Design review of the part built by this model. Coordinates are the model's own, in mm. A direction names the side the tool comes from. Coordinates: 2 decimals unless noted, no trailing zeros. Loops run counter-clockwise (first coordinate to the right, second up) from the corner with the lowest first, then second, coordinate; pieces in that order, holes last. Notation, with made-up numbers: (-31.5, 79.25) -> (-5.5, 79.25) arc R26 cw to (-5.5, 96.25) -> close; hole circle Ø3 at (64, -29). An arc over 180 degrees is marked (long way). Use one line per item in the form item = value. Start each with the question number.
1. For pin 1 (2 mm diameter, centred on x = 1, z = 27.5, fed in from -Y); pin 2 (1 mm diameter, centred on x = 0, y = 0, fed in from -Z); pin 3 (2 mm diameter, centred on x = -1.5, z = 53.5, fed in from +Y), all flat-tipped, find the tip position at first contact; note any pin that passes through.
2. Consider section A-A (x = 0). State the section outline as (y, z) points, then the cut area to 3 significant figures.
3. Machinability: for faces 4 (the face through (2.4, -4.5, 3)), 5 (the face through (0, -1, -6)), which of the approach directions +Z, -Z, +X, -X, +Y, -Y give a long, thin tool a straight path to every point of the face, cutting with its end or side? Answer none if there is none.
4. Consider section D-D (z = 55). State the section outline as (x, y) points, then the cut area to 3 significant figures.
5. Wall thickness on line 1 (Y direction, x = 0, z = -4.5); line 2 (Y direction, x = 0.75, z = -5); line 3 (Y direction, x = 0, z = 96): over which ranges is each line inside the solid? List them lowest first. Write a range as from..to.
6. The part is to be moulded in two halves that separate along X. For faces 1 (the face through (0, 0, 3)), 2 (the face through (-1.5, 0.07, 59.6)), 3 (the face through (3.3, -1.1, 0)), say which applies: released by +X, released by -X, zero draft, split by the parting line, or undercut.
7. Consider section C-C (z = -5.5). State the section outline as (x, y) points, then the cut area to 3 significant figures.
from build123d import *

# Parameters (mm, degrees)
ESQUISSE1_R             = 8.5
BOSS_EXTRU_1_DEPTH      = 10
ESQUISSE2_R             = 2.5
BOSS_EXTRU_2_DEPTH      = 157
ECHELLE2_SCALE          = 0.6
ESQUISSE5_R             = 3.25
BOSS_EXTRU_4_DEPTH      = 14
ESQUISSE6_R             = 1
ENL_V_MAT_EXTRU_1_DEPTH = 17
D_ME1_FACE_RADIUS       = 1.5
D_ME1_HEIGHT            = 1.5


with BuildPart() as part:
    # Esquisse1 → Boss.-Extru.1 (new body)
    with BuildSketch(Plane.XY):
        Circle(ESQUISSE1_R)
    extrude(amount=BOSS_EXTRU_1_DEPTH)

    # Esquisse2 → Boss.-Extru.2 (add)
    with BuildSketch(Plane.XY.offset(10)):
        Circle(ESQUISSE2_R)
    extrude(amount=BOSS_EXTRU_2_DEPTH)


with BuildPart() as part_1:
    # Echelle2: scaled about (0, 0, 0)
    add(part.part.scale(ECHELLE2_SCALE))

    # Esquisse5 → Boss.-Extru.4 (add)
    with BuildSketch(Plane(origin=(0, 0, 0), x_dir=(-1, 0, 0), z_dir=(0, 0, -1))):
        with Locations(Location((0, 0, 0), (0, 0, 180))):
            Circle(ESQUISSE5_R)
    extrude(amount=BOSS_EXTRU_4_DEPTH)

    # Esquisse6 → Enlèv. mat.-Extru.1 (cut)
    with BuildSketch(Plane(origin=(0, 0, -14), x_dir=(-1, 0, 0), z_dir=(0, 0, -1))):
        Circle(ESQUISSE6_R)
    extrude(amount=-ENL_V_MAT_EXTRU_1_DEPTH, mode=Mode.SUBTRACT)

    # Esquisse8 → Révolution1 (revolve)
    with BuildSketch(Plane(origin=(0, 0, 0), x_dir=(1, 0, 0), z_dir=(0, 1, 0)), mode=Mode.PRIVATE) as r_volution1_sk:
        Polygon((5.1, -6), (0, -6), (0, -26), align=None)
    revolve(r_volution1_sk.sketch.rotate(Axis((0, 0, 6), (0, 0, 1)), 180), axis=Axis((0, 0, 6), (0, 0, 1)))

    # Dôme1: a dome of height H over a round flat face of radius A is a cap of a sphere of radius (A * A + H * H) / (2 * H)
    d_me1_r = (D_ME1_FACE_RADIUS * D_ME1_FACE_RADIUS + D_ME1_HEIGHT * D_ME1_HEIGHT) / (2 * D_ME1_HEIGHT)
    d_me1_base = Plane((0, 0, 100.2), z_dir=(0, 0, 1))
    with Locations(d_me1_base.offset(D_ME1_HEIGHT - d_me1_r)):
        d_me1_ball = Sphere(d_me1_r, mode=Mode.PRIVATE)
    add(split(d_me1_ball, bisect_by=d_me1_base, keep=Keep.TOP, mode=Mode.PRIVATE))


solid = part_1.part
Geometry check:
q1.pin_1 = -1.5
q1.pin_2 = 3
q1.pin_3 = 1.41
q2.outline = (-5.1, 0) -> (-3.25, 0) -> (-3.25, -14) -> (-1, -14) -> (-1, 3) -> (1, 3) -> (1, -14) -> (3.25, -14) -> (3.25, 0) -> (5.1, 0) -> (5.1, 6) -> (1.5, 20.12) -> (1.5, 100.2) arc R1.5 ccw to (-1.5, 100.2) -> (-1.5, 20.12) -> (-5.1, 6) -> close
q2.area = 455 mm²
q3.face_4 = +Z, -Z
q3.face_5 = -Z
q4.outline = circle Ø3 at (0, 0)
q4.area = 7.07 mm²
q5.line_1 = -3.25..-1, 1..3.25
q5.line_2 = -3.16..-0.66, 0.66..3.16
q5.line_3 = -1.5..1.5
q6.face_1 = undercut
q6.face_2 = split by the parting line
q6.face_3 = zero draft
q7.outline = circle Ø6.5 at (0, 0); hole circle Ø2 at (0, 0)
q7.area = 30.0 mm²
